from build123d import *

# Parameters (mm, degrees)
F1_DEPTH = 2.4
F3_R     = 0.5
F4_R     = 0.2
F5_R     = 0.2
F6_R     = 0.2
F8_DEPTH = 0.6


with BuildPart() as f1:
    # F0 (on Front) → F1 (new body)
    with BuildSketch(Plane.XZ):
        with BuildLine():
            Line((1.225, 0), (0, 0))
            Line((0, 0), (0, -3.6))
            ThreePointArc((0, -3.6), (2.79331856, -2.235219763), (4.6334154242, -4.7410723531))
            Line((4.6334154242, -4.7410723531), (6.0834154242, -4.7410723531))
            Line((6.0834154242, -4.7410723531), (4.3253234554, -0.970831959))
            Line((4.3253234554, -0.970831959), (8.5253234554, -0.970831959))
            Line((8.5253234554, -0.970831959), (9.825, 2.6))
            Line((9.825, 2.6), (1.225, 2.6))
            Line((1.225, 2.6), (1.225, 0))
        make_face()
    extrude(amount=F1_DEPTH)

    # F2: F1 across face


with BuildPart() as f1_1:
    add(f1.part)
    add(f1.part.mirror(Plane(origin=(0, -1.2, -1.8), x_dir=(0, -1, 0), z_dir=(-1, 0, 0))))

    # F3
    f3_edges = [f1_1.edges().sort_by_distance(p)[0] for p in [
        (-9.825, -1.2, 2.6),
        (9.825, -1.2, 2.6),
    ]]
    fillet(f3_edges, radius=F3_R)

    # F4
    f4_edges = [f1_1.edges().sort_by_distance(p)[0] for p in [
        (-8.525323, -1.2, -0.970832),
        (8.525323, -1.2, -0.970832),
    ]]
    fillet(f4_edges, radius=F4_R)

    # F5
    f5_edges = [f1_1.edges().sort_by_distance(p)[0] for p in [
        (-6.083415, -1.2, -4.741072),
        (6.083415, -1.2, -4.741072),
    ]]
    fillet(f5_edges, radius=F5_R)

    # F6
    f6_edges = [f1_1.edges().sort_by_distance(p)[0] for p in [
        (-4.325323, -1.2, -0.970832),
        (4.325323, -1.2, -0.970832),
    ]]
    fillet(f6_edges, radius=F6_R)

    # F7 (on face) → F8 (cut)
    with BuildSketch(Plane.XZ.offset(2.4)):
        Polygon((1.725, -0.6), (-1.725, -0.6), (-1.725, 2.6), (-2.975, 2.6), (-2.975, -1.1), (2.975, -1.1), (2.975, 2.6), (1.725, 2.6), align=None)
    extrude(amount=-F8_DEPTH, mode=Mode.SUBTRACT)


solid = f1_1.part
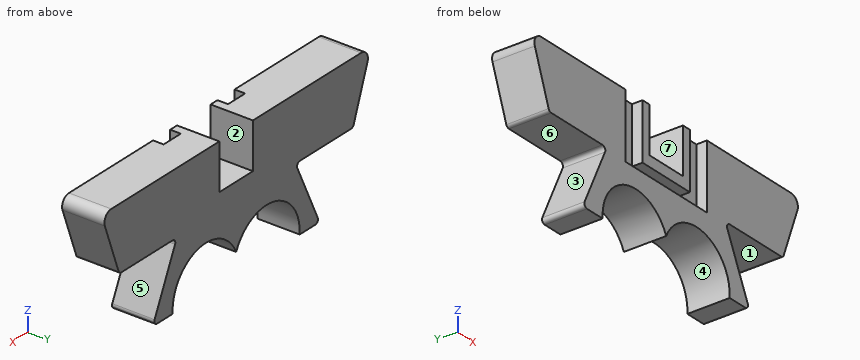
Geometry check sheet. Reference: the model listing, model coordinates, mm. Face numbers are marked on the shaded views. A direction names the side the tool comes from. Round coordinates to 2 decimals unless told otherwise and drop trailing zeros. Loops run counter-clockwise (first coordinate to the right, second up) from the corner with the lowest first, then second, coordinate; pieces in that order, holes last. Notation, with made-up numbers: (49, 3) - (93, 3) arc R27 ccw to (93, 21) - close; hole circle Ø1 at (-32.5, -21). An arc over 180 degrees is marked (long way). One line per question, with ' | ' between items. Start each with the question number.
1. Scan lines: line 1 (X direction, y = -1.25, z = -2.5); line 2 (X direction, y = -0.85, z = 2) (3 decimals); line 3 (Z direction, x = 6.5, y = -0.1). Record each from-to range of solid material in increasing order. Write a range as [from, to].
2. Cross-section at B-B on x = 5. Record the cut outline in (y, z), then the cut area to 3 significant figures.
3. Tool access check on the marked faces 5, 6 and 7. Record the directions out of +Z, -Z, +X, -X, +Y, -Y that give a thin tool (end or side, any length) a straight path to the whole face; none if there is none.
4. Draft check along X on the marked faces 1, 2, 3 and 4. Enter one of: released by +X, released by -X, zero draft, split by the parting line, or undercut.
5. Depth check by flat-ended pin: pin 1 (0.5 mm diameter, centred on y = -2, z = 1.5, fed in from +X); pin 2 (0.7 mm diameter, centred on y = -2, z = 1, fed in from -X). Enter the tip coordinate at first touch or a pass-through.
6. Cross-section at C-C on z = 0.5. Record the cut outline in (x, y) (3 decimals), then the cut area to 3 significant figures.
Taken from the geometry:
1) line 1: [-5.04, -3.44], [-0.98, 0.98], [3.44, 5.04] | line 2: [-9.601, -1.225], [1.225, 9.601] | line 3: [-0.97, 2.6]
2) outline: (-2.4, -4.74) - (0, -4.74) - (0, -2.42) - (-2.4, -2.42) - close; (-2.4, -0.97) - (0, -0.97) - (0, 2.6) - (-2.4, 2.6) - close | area: 14.1 mm²
3) face 5: +X, +Y, -Y | face 6: -X, +Y, -Y | face 7: +Z, +Y, -Y
4) face 1: zero draft | face 2: undercut | face 3: released by -X | face 4: undercut
5) pin 1: x = 9.52 | pin 2: x = -9.37
6) outline: (-9.061, -2.4) - (-2.975, -2.4) - (-2.975, -1.8) - (-1.725, -1.8) - (-1.725, -2.4) - (-1.225, -2.4) - (-1.225, 0) - (-9.061, 0) - close; (1.225, -2.4) - (1.725, -2.4) - (1.725, -1.8) - (2.975, -1.8) - (2.975, -2.4) - (9.061, -2.4) - (9.061, 0) - (1.225, 0) - close | area: 36.1 mm²
